from build123d import *

# Parameters (mm, degrees)
CYLINDER799_R               = 1.5
CYLINDER799_DEPTH           = 100
CYLINDER799_PLACEMENT_ANGLE = 100
CYLINDER797_R               = 1.5
CYLINDER797_DEPTH           = 100
CYLINDER797_PLACEMENT_ANGLE = 135
CYLINDER801_R               = 1.5
CYLINDER801_DEPTH           = 100
CYLINDER803_R               = 1.5
CYLINDER803_DEPTH           = 100
CYLINDER803_PLACEMENT_ANGLE = 225
CYLINDER796_R               = 1.5
CYLINDER796_DEPTH           = 100
CYLINDER800_R               = 1.5
CYLINDER800_DEPTH           = 100
CYLINDER800_PLACEMENT_ANGLE = 55
CYLINDER798_R               = 1.5
CYLINDER798_DEPTH           = 100
CYLINDER802_R               = 1.5
CYLINDER802_DEPTH           = 100
CYLINDER802_PLACEMENT_ANGLE = 45
CYLINDER766_R               = 8
CYLINDER766_DEPTH           = 20
CYLINDER766_PLACEMENT_ANGLE = 100
CYLINDER765_R               = 8
CYLINDER765_DEPTH           = 20
CYLINDER765_PLACEMENT_ANGLE = 135
CYLINDER767_R               = 8
CYLINDER767_DEPTH           = 20
CYLINDER762_R               = 8
CYLINDER762_DEPTH           = 20
CYLINDER762_PLACEMENT_ANGLE = 225
CYLINDER769_R               = 8
CYLINDER769_DEPTH           = 20
CYLINDER764_R               = 8
CYLINDER764_DEPTH           = 20
CYLINDER764_PLACEMENT_ANGLE = 55
CYLINDER763_R               = 8
CYLINDER763_DEPTH           = 20
CYLINDER768_R               = 8
CYLINDER768_DEPTH           = 20
CYLINDER768_PLACEMENT_ANGLE = 45
TUBE082_R                   = 58
TUBE082_R_2                 = 30
TUBE082_DEPTH               = 8


with BuildPart() as obj1:
    # Cylinder799 → Cylinder799 (new body)
    with BuildSketch(Plane.XY):
        Circle(CYLINDER799_R)
    extrude(amount=CYLINDER799_DEPTH)


with BuildPart() as obj1_1:
    # Cylinder799 placement: moved
    add(obj1.part.moved(Location((41.004432, -9.090464, 0))).rotate(Axis((41.004432, -9.090464, 0), (0, 0, 1)), CYLINDER799_PLACEMENT_ANGLE))


with BuildPart() as obj2:
    # Cylinder797 → Cylinder797 (new body)
    with BuildSketch(Plane.XY):
        Circle(CYLINDER797_R)
    extrude(amount=CYLINDER797_DEPTH)


with BuildPart() as obj2_1:
    # Cylinder797 placement: moved
    add(obj2.part.moved(Location((38.80294, 16.072704, 0))).rotate(Axis((38.80294, 16.072704, 0), (0, 0, 1)), CYLINDER797_PLACEMENT_ANGLE))


with BuildPart() as obj3:
    # Cylinder801 → Cylinder801 (new body)
    with BuildSketch(Plane(origin=(16.072704, 38.80294, 0), x_dir=(-1, 0, 0), z_dir=(0, 0, 1))):
        Circle(CYLINDER801_R)
    extrude(amount=CYLINDER801_DEPTH)


with BuildPart() as obj4:
    # Cylinder803 → Cylinder803 (new body)
    with BuildSketch(Plane.XY):
        Circle(CYLINDER803_R)
    extrude(amount=CYLINDER803_DEPTH)


with BuildPart() as obj4_1:
    # Cylinder803 placement: moved
    add(obj4.part.moved(Location((-16.072704, 38.80294, 0))).rotate(Axis((-16.072704, 38.80294, 0), (0, 0, 1)), CYLINDER803_PLACEMENT_ANGLE))


with BuildPart() as obj5:
    # Cylinder796 → Cylinder796 (new body)
    with BuildSketch(Plane(origin=(-38.80294, 16.072704, 0), x_dir=(0, -1, 0), z_dir=(0, 0, 1))):
        Circle(CYLINDER796_R)
    extrude(amount=CYLINDER796_DEPTH)


with BuildPart() as obj6:
    # Cylinder800 → Cylinder800 (new body)
    with BuildSketch(Plane.XY):
        Circle(CYLINDER800_R)
    extrude(amount=CYLINDER800_DEPTH)


with BuildPart() as obj6_1:
    # Cylinder800 placement: moved
    add(obj6.part.moved(Location((-41.004432, -9.090464, 0))).rotate(Axis((-41.004432, -9.090464, 0), (0, 0, -1)), CYLINDER800_PLACEMENT_ANGLE))


with BuildPart() as obj7:
    # Cylinder798 → Cylinder798 (new body)
    with BuildSketch(Plane(origin=(-16.072704, -38.80294, 0), x_dir=(1, 0, 0), z_dir=(0, 0, 1))):
        Circle(CYLINDER798_R)
    extrude(amount=CYLINDER798_DEPTH)


with BuildPart() as compound716:
    # Cylinder802 → Cylinder802 (new body)
    with BuildSketch(Plane.XY):
        Circle(CYLINDER802_R)
    extrude(amount=CYLINDER802_DEPTH)


with BuildPart() as compound716_1:
    # Cylinder802 placement: moved
    add(compound716.part.moved(Location((16.072704, -38.80294, 0))).rotate(Axis((16.072704, -38.80294, 0), (0, 0, 1)), CYLINDER802_PLACEMENT_ANGLE))

    # Compound716: union obj1, obj2, obj3, obj4, obj5, obj6, obj7
    add(obj1_1.part)
    add(obj2_1.part)
    add(obj3.part)
    add(obj4_1.part)
    add(obj5.part)
    add(obj6_1.part)
    add(obj7.part)


with BuildPart() as obj8:
    # Cylinder766 → Cylinder766 (new body)
    with BuildSketch(Plane.XY):
        Circle(CYLINDER766_R)
    extrude(amount=CYLINDER766_DEPTH)


with BuildPart() as obj8_1:
    # Cylinder766 placement: moved
    add(obj8.part.moved(Location((41.004432, -9.090464, 0))).rotate(Axis((41.004432, -9.090464, 0), (0, 0, 1)), CYLINDER766_PLACEMENT_ANGLE))


with BuildPart() as obj9:
    # Cylinder765 → Cylinder765 (new body)
    with BuildSketch(Plane.XY):
        Circle(CYLINDER765_R)
    extrude(amount=CYLINDER765_DEPTH)


with BuildPart() as obj9_1:
    # Cylinder765 placement: moved
    add(obj9.part.moved(Location((38.80294, 16.072704, 0))).rotate(Axis((38.80294, 16.072704, 0), (0, 0, 1)), CYLINDER765_PLACEMENT_ANGLE))


with BuildPart() as obj10:
    # Cylinder767 → Cylinder767 (new body)
    with BuildSketch(Plane(origin=(16.072704, 38.80294, 0), x_dir=(-1, 0, 0), z_dir=(0, 0, 1))):
        Circle(CYLINDER767_R)
    extrude(amount=CYLINDER767_DEPTH)


with BuildPart() as obj11:
    # Cylinder762 → Cylinder762 (new body)
    with BuildSketch(Plane.XY):
        Circle(CYLINDER762_R)
    extrude(amount=CYLINDER762_DEPTH)


with BuildPart() as obj11_1:
    # Cylinder762 placement: moved
    add(obj11.part.moved(Location((-16.072704, 38.80294, 0))).rotate(Axis((-16.072704, 38.80294, 0), (0, 0, 1)), CYLINDER762_PLACEMENT_ANGLE))


with BuildPart() as obj12:
    # Cylinder769 → Cylinder769 (new body)
    with BuildSketch(Plane(origin=(-38.80294, 16.072704, 0), x_dir=(0, -1, 0), z_dir=(0, 0, 1))):
        Circle(CYLINDER769_R)
    extrude(amount=CYLINDER769_DEPTH)


with BuildPart() as obj13:
    # Cylinder764 → Cylinder764 (new body)
    with BuildSketch(Plane.XY):
        Circle(CYLINDER764_R)
    extrude(amount=CYLINDER764_DEPTH)


with BuildPart() as obj13_1:
    # Cylinder764 placement: moved
    add(obj13.part.moved(Location((-41.004432, -9.090464, 0))).rotate(Axis((-41.004432, -9.090464, 0), (0, 0, -1)), CYLINDER764_PLACEMENT_ANGLE))


with BuildPart() as obj14:
    # Cylinder763 → Cylinder763 (new body)
    with BuildSketch(Plane(origin=(-16.072704, -38.80294, 0), x_dir=(1, 0, 0), z_dir=(0, 0, 1))):
        Circle(CYLINDER763_R)
    extrude(amount=CYLINDER763_DEPTH)


with BuildPart() as compound710:
    # Cylinder768 → Cylinder768 (new body)
    with BuildSketch(Plane.XY):
        Circle(CYLINDER768_R)
    extrude(amount=CYLINDER768_DEPTH)


with BuildPart() as compound710_1:
    # Cylinder768 placement: moved
    add(compound710.part.moved(Location((16.072704, -38.80294, 0))).rotate(Axis((16.072704, -38.80294, 0), (0, 0, 1)), CYLINDER768_PLACEMENT_ANGLE))

    # Compound710: union obj8, obj9, obj10, obj11, obj12, obj13, obj14
    add(obj8_1.part)
    add(obj9_1.part)
    add(obj10.part)
    add(obj11_1.part)
    add(obj12.part)
    add(obj13_1.part)
    add(obj14.part)


with BuildPart() as compound710_2:
    # Compound710 placement: moved
    add(compound710_1.part.moved(Location((0, 0, 56))))


with BuildPart() as cut333:
    # Tube082 → Tube082 (new body)
    with BuildSketch(Plane.XY.offset(52)):
        Circle(TUBE082_R)
        Circle(TUBE082_R_2, mode=Mode.SUBTRACT)
    extrude(amount=TUBE082_DEPTH)

    # Cut332: cut Compound710
    add(compound710_2.part, mode=Mode.SUBTRACT)

    # Cut333: cut Compound716
    add(compound716_1.part, mode=Mode.SUBTRACT)


solid = cut333.part
Model file for the job. Use its own axes, mm. A direction names the side the tool comes from. Give positions to 0.01 mm unless a question says otherwise; leave off trailing zeros. Loops run counter-clockwise (first coordinate to the right, second up) from the corner with the lowest first, then second, coordinate; pieces in that order, holes last.
Item 1: Drop flat-ended pins along their axis: P1, Ø2.5, axis at x = -41, y = -9.09, coming from the +Z side; P2, Ø2, axis at x = 2, z = 54.5, coming from the -Y side; P3, Ø14.5, axis at x = -16.07, y = 38.8, coming from the +Z side; P4, Ø3, axis at x = 13, z = 56.5, coming from the +Y side. Give the stop position or say it passes through.
Check values:
P1: passes through
P2: stops at y = -57.99
P3: stops at z = 56
P4: stops at y = 56.85
Item 2: Slice it at A-A (y = -25). Write the cut outline in (x, z).
Check values:
outline: (-52.34, 52) - (-16.58, 52) - (-16.58, 60) - (-52.34, 60) - close; (16.58, 52) - (52.34, 52) - (52.34, 60) - (16.58, 60) - close
Item 3: Slice it at D-D (y = -6). Write the cut outline in (x, z).
Check values:
outline: (-57.69, 52) - (-29.39, 52) - (-29.39, 60) - (-33.63, 60) - (-33.63, 56) - (-48.38, 56) - (-48.38, 60) - (-57.69, 60) - close; (29.39, 52) - (57.69, 52) - (57.69, 60) - (48.38, 60) - (48.38, 56) - (33.63, 56) - (33.63, 60) - (29.39, 60) - close
Item 4: Mould opens along Y. For faces 1 (the face through (25, -25, 52)), 2 (the face through (40.1, 17.2, 56)) say: +Y half, -Y half, draft (parallel to the pull), parting line (faces both ways), or undercut.
Check values:
face 1: draft
face 2: undercut
Item 5: Slice it at B-B (x = 0). Write the cut outline in (y, z).
Check values:
outline: (-58, 52) - (-30, 52) - (-30, 60) - (-58, 60) - close; (30, 52) - (58, 52) - (58, 60) - (30, 60) - close
Item 6: Drill centre lines: line 1 along X through (y, z) = (0.5, 58.25); line 2 along Y through (x, z) = (-22, 57.5); line 3 along X through (y, z) = (-43.5, 57.25). Where is each one in solid material? Low to high.
Check values:
line 1: x = -58 to -30, 30 to 58
line 2: y = -53.67 to -44.18, -33.43 to -20.4, 20.4 to 33.43, 44.18 to 53.67
line 3: x = -38.36 to -22.55, -9.6 to 9.6, 22.55 to 38.36
Item 7: Which spindle directions (+Z, -Z, +X, -X, +Y, -Y) get a long thin tool onto all of the face, cutting with end or side? Do faces 3 (the face through (-8.442, -36.4, 57.972)), 4 (the face through (-37.538, 15.266, 53.972)). Say none if no direction does.
Check values:
face 3: +Z
face 4: +Z, -Z
Item 8: Slice it at C-C (z = 57.75). Give the number of separate pieces and of enclosed holes in the cut face, plus the area to 3 significant figures.
Check values:
separate pieces: 1
enclosed holes: 9
area: 6,130 mm2
